Work out the finished part from the listing and answer in its coordinate system (mm). A direction names the side the tool comes from. Round coordinates to 2 decimals unless told otherwise and drop trailing zeros. Write each loop counter-clockwise with the first axis right and the second up, starting at its lowest first coordinate (ties: lowest second). Pieces come first, ordered by that corner, then holes. Notation, with made-up numbers: (12.5, 9) - (71.5, 9) arc R30 cw to (71.5, 44) - close; hole circle Ø1 at (16, 81). An arc over 180 degrees is marked (long way). Answer as a JSON object with one key per item and string values.
```python
from build123d import *

# Parameters (mm, degrees)
SKETCH_1_W          = 20
SKETCH_1_H          = 20
SKETCH_1_W_2        = 18
SKETCH_1_H_2        = 18
EXTRUDE_1_DEPTH     = 55
SKETCH_3_R          = 2.05
SKETCH_3_R_2        = 3.05
CUT_EXTRUDE_1_DEPTH = 20
SKETCH_4_R          = 2.05
SKETCH_4_R_2        = 3.025
CUT_EXTRUDE_2_DEPTH = 60.371710435
SKETCH_5_R          = 2.05
CUT_EXTRUDE_3_DEPTH = 30


with BuildPart() as part:
    # 草图1 → 凸台-拉伸1 (new, symmetric)
    with BuildSketch(Plane.XY):
        Rectangle(SKETCH_1_W, SKETCH_1_H)
        Rectangle(SKETCH_1_W_2, SKETCH_1_H_2, mode=Mode.SUBTRACT)
    extrude(amount=EXTRUDE_1_DEPTH, both=True)

    # 草图3 → 切除-拉伸1 (cut)
    with BuildSketch(Plane(origin=(0, 10, 0), x_dir=(1, 0, 0), z_dir=(0, 1, 0))):
        with Locations(Location((-5, -31, 0), (0, 0, 270))):
            Circle(SKETCH_3_R)
        with Locations(Location((5, -31, 0), (0, 0, 270))):
            Circle(SKETCH_3_R)
        with Locations(Location((5, -51, 0), (0, 0, 270))):
            Circle(SKETCH_3_R)
        with Locations(Location((-5, -51, 0), (0, 0, 270))):
            Circle(SKETCH_3_R)
        with Locations(Location((0, -41, 0), (0, 0, 270))):
            Circle(SKETCH_3_R_2)
    extrude(amount=-CUT_EXTRUDE_1_DEPTH, mode=Mode.SUBTRACT)

    # 草图4 → 切除-拉伸2 (cut, through all)
    with BuildSketch(Plane.XZ.offset(10)):
        with Locations(Location((0, -51, 0), (0, 0, 270))):
            Circle(SKETCH_4_R)
        with Locations(Location((0, -31, 0), (0, 0, 270))):
            Circle(SKETCH_4_R)
        with Locations(Location((0, -41, 0), (0, 0, 270))):
            Circle(SKETCH_4_R_2)
    extrude(amount=-CUT_EXTRUDE_2_DEPTH, mode=Mode.SUBTRACT)

    # 草图5 → 切除-拉伸3 (cut)
    with BuildSketch(Plane(origin=(10, 0, 0), x_dir=(0, 0, -1), z_dir=(1, 0, 0))):
        with Locations((-50, 0)):
            Circle(SKETCH_5_R)
        with Locations((-40, 0)):
            Circle(SKETCH_5_R)
        with Locations((-30, 0)):
            Circle(SKETCH_5_R)
        with Locations((-20, 0)):
            Circle(SKETCH_5_R)
        with Locations((-10, 0)):
            Circle(SKETCH_5_R)
        Circle(SKETCH_5_R)
        with Locations((10, 0)):
            Circle(SKETCH_5_R)
        with Locations((20, 0)):
            Circle(SKETCH_5_R)
        with Locations((30, 0)):
            Circle(SKETCH_5_R)
        with Locations((40, 0)):
            Circle(SKETCH_5_R)
        with Locations((50, 0)):
            Circle(SKETCH_5_R)
    extrude(amount=-CUT_EXTRUDE_3_DEPTH, mode=Mode.SUBTRACT)


solid = part.part
```
Item 1: A cutting plane is placed at A-A (z = -10). Write down the section's boundary in (x, y).
Results found:
{"outline": "(-10, -10) - (10, -10) - (10, -2.05) - (9, -2.05) - (9, -9) - (-9, -9) - (-9, -2.05) - (-10, -2.05) - close; (-10, 2.05) - (-9, 2.05) - (-9, 9) - (9, 9) - (9, 2.05) - (10, 2.05) - (10, 10) - (-10, 10) - close"}
Item 2: A cutting plane is placed at C-C (x = 5). Write down the section's boundary in (y, z).
Results found:
{"outline": "(-10, -55) - (-9, -55) - (-9, 28.95) - (-10, 28.95) - close; (-10, 33.05) - (-9, 33.05) - (-9, 48.95) - (-10, 48.95) - close; (-10, 53.05) - (-9, 53.05) - (-9, 55) - (-10, 55) - close; (9, -55) - (10, -55) - (10, 28.95) - (9, 28.95) - close; (9, 33.05) - (10, 33.05) - (10, 48.95) - (9, 48.95) - close; (9, 53.05) - (10, 53.05) - (10, 55) - (9, 55) - close"}
Item 3: A cutting plane is placed at B-B (y = -5). Write down the section's boundary in (x, z), and give its area (3 significant figures).
Results found:
{"outline": "(-10, -55) - (-9, -55) - (-9, 55) - (-10, 55) - close; (9, -55) - (10, -55) - (10, 55) - (9, 55) - close", "area": "220 mm²"}
Item 4: A cutting plane is placed at D-D (z = -23). Write down the section's boundary in (x, y), and give its area (3 significant figures).
Results found:
{"outline": "(-10, -10) - (10, -10) - (10, 10) - (-10, 10) - close; hole (-9, -9) - (9, -9) - (9, 9) - (-9, 9) - close", "area": "76.0 mm²"}
Item 5: For faces 3 (the cylindrical face through (-9.49, 0.09, 12.05)), 4 (the flat face through (9, -2, 1)), determine the directions among +Z, -Z, +X, -X, +Y, -Y from which every point of the face is accessible in a straight line to the end or side of a thin tool.
Results found:
{"face 3": "+X, -X", "face 4": "+Z, -Z"}
Item 6: Consider line 1 along Y through (x, z) = (-4, 1); line 2 along Y through (x, z) = (-9.3, 10). Determine where each line is inside the solid, lowest interval first.
Results found:
{"line 1": "-10 to -9, 9 to 10", "line 2": "-10 to -2.05, 2.05 to 10"}
Item 7: Determine the mould class of faces 1 (the cylindrical face through (5.09, 9.51, 28.95)), 2 (the flat face through (10, -2, 1)) for opening direction Z: pulls with the +Z half, pulls with the -Z half, needs draft (parallel to the pull), parting line crosses it, or undercut.
Results found:
{"face 1": "undercut", "face 2": "needs draft"}
